Work out the finished part from the listing and answer in its coordinate system (mm). Coordinates: 2 decimals unless noted, no trailing zeros. Write each question's results on one line, items separated by ' | '. Start each with the question number.
1. Find the intervals of material crossed by line 1 along Y through (x, z) = (305, 1.5); line 2 along X through (y, z) = (-29, 2.15); line 3 along X through (y, z) = (172, 1.6), in increasing order. Write a range as [from, to].
2. This flat-tipped pin is pushed along its axis until it touches: P1, Ø7, axis at x = -293, y = -124, coming from the +Z side. Where does it stop, or does it pass through?
3. Determine the mould class of faces 1 (the cylindrical face through (299.5, 225.1, 3.5)), 2 (the cylindrical face through (269.032, -213.676, 3.47)) for opening direction Y: released by +Y, released by -Y, zero draft, split by the parting line, or undercut.
from build123d import *

# Parameters (mm, degrees)
F0_W           = 750
F0_H           = 500
F1_DEPTH       = 5
F4_D           = 9
F4_CBORE_D     = 15
F4_CBORE_DEPTH = 3
F3_W           = 235
F3_H           = 240
F5_DEPTH       = 0.1
F6_DEPTH       = 0.1
F3_W_2         = 59
F3_H_2         = 112
F7_DEPTH       = 0.1
F8_DEPTH       = 0.1
F9_DEPTH       = 0.1
F11_D          = 4.4
F12_D          = 5.5
F13_D          = 6.6
F15_D          = 20
F16_W          = 36
F16_H          = 30
F16_W_2        = 30
F16_H_2        = 36
F17_DEPTH      = 0.1


# Not quite as in the source:
# - a feature names something its author has since deleted; it is built from what else it names


with BuildPart() as f1:
    # F0 (on Top) → F1 (new body)
    with BuildSketch(Plane.XY):
        Rectangle(F0_W, F0_H)
    extrude(amount=F1_DEPTH)

    # F4 (through all)
    with Locations(Plane.XY.offset(5)):
        with Locations((-305, 220), (-265, 220), (-305, -220), (-265, -220), (265, -220), (305, -220), (265, 220), (305, 220)):
            CounterBoreHole(F4_D / 2, F4_CBORE_D / 2, F4_CBORE_DEPTH)

    # F3 (on face) → F5 (cut)
    with BuildSketch(Plane.XY.offset(5)):
        with Locations((232.5, -120)):
            Rectangle(F3_W, F3_H)
    extrude(amount=-F5_DEPTH, mode=Mode.SUBTRACT)

    # F3 (on face) → F6 (cut)
    with BuildSketch(Plane.XY.offset(5)):
        Polygon((180, 122.1947473288), (180, 165), (180, 185), (55, 185), (55, 145), (55, 105), (180, 105), align=None)
    extrude(amount=-F6_DEPTH, mode=Mode.SUBTRACT)

    # F3 (on face) → F7 (cut)
    with BuildSketch(Plane.XY.offset(5)):
        with Locations((-285.5, -129)):
            Rectangle(F3_W_2, F3_H_2)
    extrude(amount=-F7_DEPTH, mode=Mode.SUBTRACT)

    # F3 (on face) → F8 (cut)
    with BuildSketch(Plane.XY.offset(5)):
        Polygon((35, 230), (-205, 230), (-205, 190), (35, 190), (35, 210), align=None)
    extrude(amount=-F8_DEPTH, mode=Mode.SUBTRACT)

    # F3 (on face) → F9 (cut)
    with BuildSketch(Plane.XY.offset(5)):
        Polygon((-208.5, -108), (-221, -108), (-221, -185), (-196, -185), (-196, -108), align=None)
        Polygon((-136, -185), (-136, -108), (-148.5, -108), (-161, -108), (-161, -185), align=None)
        Polygon((-76, -185), (-76, -108), (-88.5, -108), (-101, -108), (-101, -185), align=None)
        Polygon((-16, -185), (-16, -108), (-28.5, -108), (-41, -108), (-41, -185), align=None)
        Polygon((31.5, -108), (19, -108), (19, -185), (44, -185), (44, -108), align=None)
    extrude(amount=-F9_DEPTH, mode=Mode.SUBTRACT)

    # F11 (through all)
    with Locations(Plane.XY.offset(5)):
        with Locations((-285.5, -134), (-293, -124), (-278, -78), (-285.5, -180), (-216, -180), (-201, -113), (-141, -113), (-156, -180), (-96, -180), (-81, -113), (-21, -113), (-36, -180), (24, -180), (39, -113)):
            Hole(F11_D / 2)

    # F12 (through all)
    with Locations(Plane.XY.offset(5)):
        with Locations((-190, 220), (-190, 200), (20, 200), (20, 220)):
            Hole(F12_D / 2)

    # F13 (through all)
    with Locations(Plane.XY.offset(5)):
        with Locations((60, 118), (175, 172), (102, -30), (102, -210), (363, -210), (363, -30)):
            Hole(F13_D / 2)

    # F15 (through all)
    with Locations(Plane.XY.offset(5)):
        with Locations((-303.5, 38)):
            Hole(F15_D / 2)

    # F16 (on face) → F17 (cut)
    with BuildSketch(Plane.XY.offset(5)):
        with Locations((-348.5, -10)):
            Rectangle(F16_W, F16_H)
        with Locations((-350, 145)):
            Rectangle(F16_W_2, F16_H_2)
        with Locations((-240, 145)):
            Rectangle(F16_W_2, F16_H_2)
    extrude(amount=-F17_DEPTH, mode=Mode.SUBTRACT)


solid = f1.part
Values:
1) line 1: [-250, -224.5], [-215.5, 215.5], [224.5, 250] | line 2: [-375, 98.86], [105.14, 359.86], [366.14, 375] | line 3: [-375, 171.7], [178.3, 375]
2) P1: z = 4.9
3) face 1: undercut | face 2: undercut
